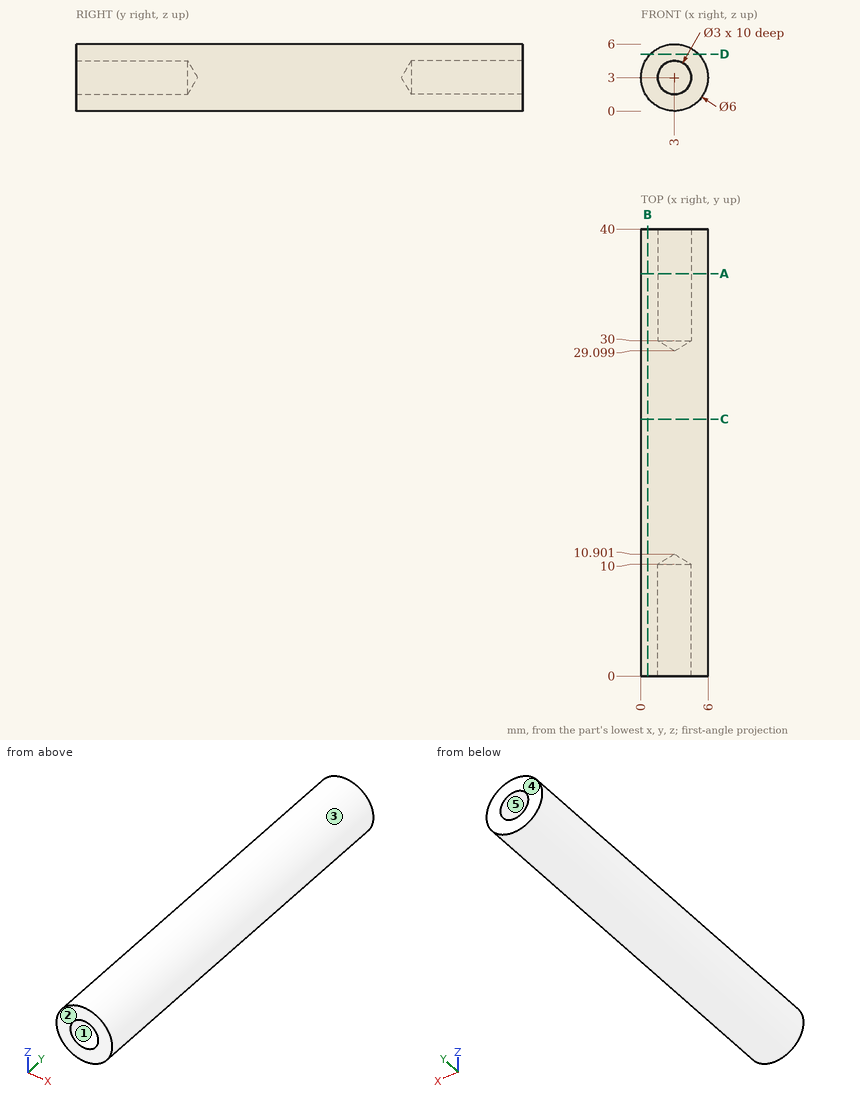
For this review, use the dimensioned drawing (mm, ordinates from the lowest corner) and the shaded views. A direction names the side the tool comes from. Give positions to 0.01 mm unless a question says otherwise; leave off trailing zeros. Order: outer loops, then holes, each group sorted by start corner. A loop starts at its lowest first (then second) coordinate and runs counter-clockwise, first axis right, second up. Notation, with made-up numbers: (-5, 54.5) -> (39, 54.5) arc R22 cw to (39, 72.5) -> close; hole circle Ø8 at (-22.5, 79). An arc over 180 degrees is marked (long way). Write item = value, one per line. Start each with the question number.
(1) Take a section at C-C (y = 23). Write out the cut boundary in (x, z).
(2) Draft analysis for pull direction X (two halves, no side actions). For the marked faces 3, 4 and 5, state which applies: +X half, -X half, draft (parallel to the pull), parting line (faces both ways), or undercut.
(3) Take a section at D-D (z = 5.1). Write out the cut boundary in (x, y).
(4) Tool access review of the marked faces 1 and 2: name each direction out of +Z, -Z, +X, -X, +Y, -Y from which nothing blocks a thin tool from reaching the whole face with its end or side.
(5) For L1, parallel to X at y = 5.25, z = 3; L2, parallel to Z at x = 3.7, y = 8, list the stretches that pass through material, from the lowest coordinate up. Write a range as from..to.
(6) Take a section at A-A (y = 36). Write out the cut boundary in (x, z).
(7) Take a section at B-B (x = 0.6). Write out the cut boundary in (y, z).
Returned:
q1.outline = circle Ø6 at (3, 3)
q2.face_3 = parting line
q2.face_4 = draft
q2.face_5 = undercut
q3.outline = (0.86, 0) -> (5.14, 0) -> (5.14, 40) -> (0.86, 40) -> close
q4.face_1 = -Y
q4.face_2 = +Z, -Z, +X, -X, -Y
q5.L1 = 0..1.5, 4.5..6
q5.L2 = 0.08..1.67, 4.33..5.92
q6.outline = circle Ø6 at (3, 3); hole circle Ø3 at (3, 3)
q7.outline = (0, 1.2) -> (40, 1.2) -> (40, 4.8) -> (0, 4.8) -> close
